```python
from build123d import *


# Not quite as in the source:
# - ends of sketch curves that miss each other by under 0.0002 mm in the source are joined
# - the dataset's text gives a spline's control points without its knots; the knots are read off the source's solid


with BuildPart() as f1:
    # F0 (on Front) → F1 (revolve)
    with BuildSketch(Plane.XZ):
        with BuildLine():
            Line((37.4922007322, 0), (39.4921973348, 0))
            Line((39.4921973348, 0), (39.4921973348, 10.6321773492))
            add(Edge.make_bspline(
                [(39.4921973348, 10.6321773492), (25.8319638669, 9.223905392), (-17.5490600107, 43.4075947851), (-33.0458087847, 43.4075947851)],
                knots=[0, 0, 0, 0, 79.598934163, 79.598934163, 79.598934163, 79.598934163], degree=3))
            Line((-33.0458087847, 43.4075947851), (-234.167508781, 43.4075947851))
            Line((-234.167508781, 43.4075947851), (-234.167508781, 0))
            Line((-234.167508781, 0), (-232.1675121784, 0))
            Line((-232.1675121784, 0), (-232.1675121784, 41.4075981826))
            Line((-232.1675121784, 41.4075981826), (-33.0458087847, 41.4075981826))
            add(Edge.make_bspline(
                [(37.4922013196, 8.6412238335), (37.0945770822, 8.6758484487), (35.5138249558, 8.8768940457), (32.5543086746, 9.6271891204), (28.3485189273, 11.2022557551), (22.229588287, 13.9850146115), (13.76876914, 18.4938124906), (2.9175771692, 24.7537479723), (-7.9699760264, 31.0509027544), (-16.502875169, 35.6449766342), (-22.6377369359, 38.5118930501), (-26.788697304, 40.1529468803), (-30.3678361719, 41.1839581397), (-32.2610835082, 41.4075981826), (-33.0458087847, 41.4075981826)],
                knots=[0.0410074938, 0.0410074938, 0.0410074938, 0.0410074938, 0.0625, 0.125, 0.1875, 0.25, 0.375, 0.5, 0.625, 0.75, 0.8125, 0.875, 0.9375, 1, 1, 1, 1], degree=3))
            Line((37.4922013196, 8.6412238335), (37.4922007322, 0))
        make_face()
    revolve(axis=Axis((-25.0741094351, 0, 0), (1, 0, 0)))


solid = f1.part
```
Can you work these out from the model? Positions are in its coordinate system, mm. A direction names the side the tool comes from. Give positions to 0.01 mm unless a question says otherwise; leave off trailing zeros. Order: outer loops, then holes, each group sorted by start corner. A loop starts at its lowest first (then second) coordinate and runs counter-clockwise, first axis right, second up. Notation, with made-up numbers: (-2, 3) - (21, 3) arc R21 ccw to (21, 20) - close; hole circle Ø7 at (-34, 41.5). An arc over 180 degrees is marked (long way). Use a Markdown table: item, result. Add a question column.
Q1. On a 3-axis mill with a long thin cutter (end or side, diameter ignored), from which of +Z, -Z, +X, -X, +Y, -Y can I reach the whole of each face in a straight line? I mean faces 4 (the cylindrical face through (-131.213, 40.423, -8.976)), 5 (the flat face through (-234.168, -1, -1)). Say none if no direction works.
Q2. Please list where these lines run through material, in increasing order: line 1 along Y through (x, z) = (-66, -0.5); line 2 along Z through (x, y) = (-83, 0); line 3 along X through (y, z) = (-5.5, -2).
Q3. If we mould it in two halves opening along Z, with no side actions, what happens to faces 1 (the flat face through (39.492, 0, 0)), 2 (the flat face through (-232.168, -1, 1)), 3 (the cylindrical face through (-135.015, 42.375, -9.41))? For each: released by +Z, released by -Z, zero draft, split by the parting line, or undercut.
Q4. If we section it at A-A on x = -118: Write out the boundary of the cut face in (y, z).
Q5. I'm going to push flat-ended pins straight in: pin 1 (12 mm diameter, centred on x = -80, z = 15, fed in from +Y); pin 2 (12 mm diameter, centred on x = 9.5, y = 1, fed in from -Z); pin 3 (5 mm diameter, centred on x = -187.5, y = -5.5, fed in from -Z). Where does each tip first touch, or does it pass through?
Answers follow:
| question | item | result |
|---|---|---|
| 1 | face 4 | none |
| 1 | face 5 | +Z, -Z, -X, +Y, -Y |
| 2 | line 1 | y = -43.4 to -41.4, 41.4 to 43.4 |
| 2 | line 2 | z = -43.41 to -41.41, 41.41 to 43.41 |
| 2 | line 3 | x = -234.17 to -232.17, 37.49 to 39.49 |
| 3 | face 1 | zero draft |
| 3 | face 2 | undercut |
| 3 | face 3 | split by the parting line |
| 4 | outline | circle Ø86.82 at (0, 0); hole circle Ø82.82 at (0, 0) |
| 5 | pin 1 | stops at y = 42.46 |
| 5 | pin 2 | stops at z = -26.72 |
| 5 | pin 3 | stops at z = -43.3 |
